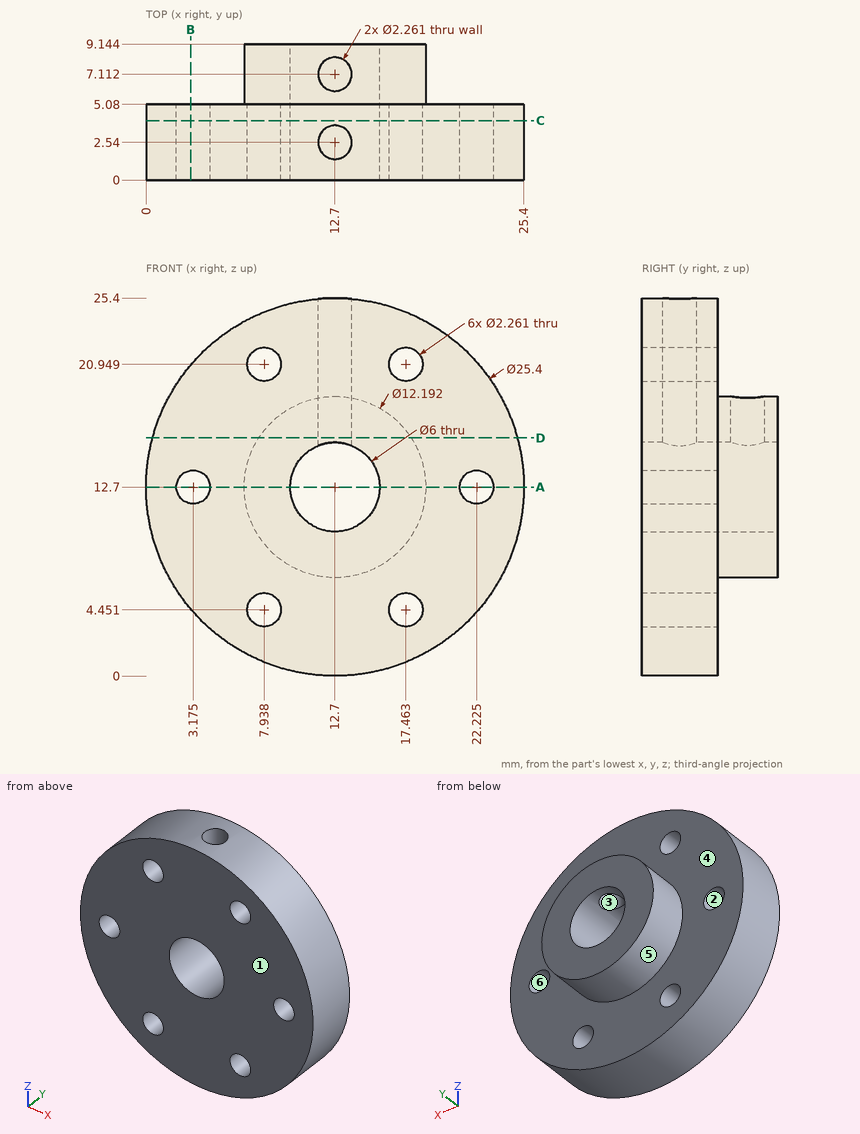
The drawing under review shows one solid part. Ordinate dimensions are in mm from its lowest x, y, z. A direction names the side the tool comes from. Round coordinates to 2 decimals unless told otherwise and drop trailing zeros. Loops run counter-clockwise (first coordinate to the right, second up) from the corner with the lowest first, then second, coordinate; pieces in that order, holes last. Notation, with made-up numbers: (35.5, 32.5) - (68.5, 32.5) arc R22 ccw to (68.5, 71.5) - close; hole circle Ø6 at (48, 87.5). An arc over 180 degrees is marked (long way). Put each result on its own line as item: value. Start each with the question number.
1. Consider section C-C on y = 4. State the section outline as (x, z) points (1 decimal), plus the area to 3 significant figures.
2. Consider section A-A on z = 12.7. State the section outline as (x, y) points (1 decimal).
3. Consider section B-B on x = 3. State the section outline as (y, z) points.
4. Insertion check: P1, Ø5, axis at y = 6.5, z = 5.5, coming from the -X side; P2, Ø5, axis at x = 5, y = 8, coming from the +Z side; P3, Ø2.5, axis at x = 7.94, z = 4.45, coming from the +Y side. Each pin has a flat end and moves straight along its axis. Give the tip position at first contact, or say it passes through.
5. Mouldability with a two-part tool opening along Y and no side actions: class the marked faces 1, 2, 3 and 4 as +Y half, -Y half, draft (parallel to the pull), parting line (faces both ways), or undercut.
6. Consider section D-D on z = 16. State the section outline as (x, y) points (1 decimal).
7. For the marked faces 5 and 6, list the 3-axis set-ups (+Z, -Z, +X, -X, +Y, -Y) from which the entire face can be reached by the end or side of a thin tool; tool diameter is ignored.
8. For probe 1 along Z at (x, y) = (7.5, 5) (1 decimal); probe 2 along Y at (x, z) = (20.5, 22.5); probe 3 along X at (y, z) = (7.25, 12.5), list the stretches that pass through material, from the lowest coordinate up. Write a range as [from, to].
Result sheet:
1. outline: circle Ø25.4 at (12.7, 12.7); hole circle Ø2.3 at (3.2, 12.7); hole circle Ø2.3 at (7.9, 4.5); hole circle Ø2.3 at (7.9, 20.9); hole circle Ø6 at (12.7, 12.7); hole circle Ø2.3 at (17.5, 4.5); hole circle Ø2.3 at (17.5, 20.9); hole circle Ø2.3 at (22.2, 12.7)
1. area: 454 mm^2
2. outline: (0, 0) - (2, 0) - (2, 5.1) - (0, 5.1) - close; (4.3, 0) - (9.7, 0) - (9.7, 9.1) - (6.6, 9.1) - (6.6, 5.1) - (4.3, 5.1) - close; (15.7, 0) - (21.1, 0) - (21.1, 5.1) - (18.8, 5.1) - (18.8, 9.1) - (15.7, 9.1) - close; (23.4, 0) - (25.4, 0) - (25.4, 5.1) - (23.4, 5.1) - close
3. outline: (0, 4.5) - (5.08, 4.5) - (5.08, 11.58) - (0, 11.58) - close; (0, 13.82) - (5.08, 13.82) - (5.08, 20.9) - (0, 20.9) - close
4. P1: x = 1.09
4. P2: z = 15.88
4. P3: y = 5.08
5. face 1: -Y half
5. face 2: draft
5. face 3: undercut
5. face 4: +Y half
6. outline: (0.4, 0) - (25, 0) - (25, 5.1) - (17.8, 5.1) - (17.8, 9.1) - (7.6, 9.1) - (7.6, 5.1) - (0.4, 5.1) - close; hole circle Ø2.3 at (12.7, 2.5); hole circle Ø2.3 at (12.7, 7.1)
7. face 5: +Y
7. face 6: +Y, -Y
8. probe 1: [1.1, 3.4], [5.5, 19.9], [22, 24.3]
8. probe 2: [0, 5.08]
8. probe 3: [6.61, 9.71], [15.69, 18.79]
